Input: part model. Units: mm. Frame: model coordinates. A direction names the side the tool comes from. Give positions to 0.01 mm unless a question says otherwise; leave off trailing zeros. Write each loop counter-clockwise with the first axis right and the second up, starting at its lowest first coordinate (ties: lowest second). Pieces come first, ordered by that corner, then holes.
```python
from build123d import *

# Parameters (mm, degrees)
F0_W           = 80
F0_H           = 50
F0_R           = 19
F0_R_2         = 11
F1_DEPTH       = 15
F2_W           = 1
F2_H           = 15
F3_DEPTH       = 25
F5_D           = 5.5
F5_DEPTH       = 18
F5_CBORE_D     = 10
F5_CBORE_DEPTH = 5
F5_TIP         = 1.6523667023
F7_D           = 5.5
F7_DEPTH       = 15
F7_TIP         = 1.6523667023
F9_D           = 5.5
F9_DEPTH       = 15
F9_TIP         = 1.6523667023
F11_D          = 5.5
F11_DEPTH      = 15
F11_TIP        = 1.6523667023
F13_D          = 5.5
F13_DEPTH      = 10
F13_TIP        = 1.6523667023


with BuildPart() as f1:
    # F0 (on Top) → F1 (new body)
    with BuildSketch(Plane.XY):
        Rectangle(F0_W, F0_H)
        with Locations((-16, 0)):
            Circle(F0_R, mode=Mode.SUBTRACT)
        with Locations((24, 0)):
            Circle(F0_R_2, mode=Mode.SUBTRACT)
    extrude(amount=F1_DEPTH)

    # F2 (on face) → F3 (cut)
    with BuildSketch(Plane.XY.offset(15)):
        with Locations((23.5, -17.5)):
            Rectangle(F2_W, F2_H)
    extrude(amount=-F3_DEPTH, mode=Mode.SUBTRACT)

    # F5
    with Locations(Plane.YZ.offset(40)):
        with Locations((-17, 7.5)):
            CounterBoreHole(F5_D / 2, F5_CBORE_D / 2, F5_CBORE_DEPTH, depth=F5_DEPTH)
            with Locations((0, 0, -(F5_DEPTH + F5_TIP / 2))):  # 118° drill point
                Cone(0, F5_D / 2, F5_TIP, mode=Mode.SUBTRACT)

    # F7
    with Locations(Plane.YZ.offset(23)):
        with Locations((-17, 7.5)):
            Hole(F7_D / 2, depth=F7_DEPTH)
            with Locations((0, 0, -(F7_DEPTH + F7_TIP / 2))):  # 118° drill point
                Cone(0, F7_D / 2, F7_TIP, mode=Mode.SUBTRACT)

    # F9
    with Locations(Plane.XZ.offset(25)):
        with Locations((-16, 7.5)):
            Hole(F9_D / 2, depth=F9_DEPTH)
            with Locations((0, 0, -(F9_DEPTH + F9_TIP / 2))):  # 118° drill point
                Cone(0, F9_D / 2, F9_TIP, mode=Mode.SUBTRACT)

    # F11
    with Locations(Plane(origin=(-40, 0, 0), x_dir=(0, -1, 0), z_dir=(-1, 0, 0))):
        with Locations((0, 7.5)):
            Hole(F11_D / 2, depth=F11_DEPTH)
            with Locations((0, 0, -(F11_DEPTH + F11_TIP / 2))):  # 118° drill point
                Cone(0, F11_D / 2, F11_TIP, mode=Mode.SUBTRACT)

    # F13
    with Locations(Plane(origin=(0, 25, 0), x_dir=(-1, 0, 0), z_dir=(0, 1, 0))):
        with Locations((-32, 7.5), (-12, 7.5)):
            Hole(F13_D / 2, depth=F13_DEPTH)
            with Locations((0, 0, -(F13_DEPTH + F13_TIP / 2))):  # 118° drill point
                Cone(0, F13_D / 2, F13_TIP, mode=Mode.SUBTRACT)


solid = f1.part
```
Q1. Section B-B, the plane z = 1. Return the cut outline in (x, y), then the cut area to 3 significant figures.
Q2. Pin query (flat end, axial travel): pin 1 (6 mm diameter, centred on y = -16.5, z = 8, fed in from +X). Return the tip coordinate at first contact, or that it passes through.
Q3. Section A-A, the plane x = -16. Return the cut outline in (y, z), then the cut area to 3 significant figures.
Q4. Access query for faces 1 (the flat face through (-1, 25, 7)), 2 (the cylindrical face through (-13.818, -21.857, 5.827)), 3 (the cylindrical face through (-37.361, -0.596, 4.815)), 4 (the cylindrical face through (13.27, 19.93, 5.06)), 5 (the cylindrical face through (29.423, -14.818, 5.827)). Directions: +Z, -Z, +X, -X, +Y, -Y. A direction counts if a zero-diameter tool reaches every point of the face in a straight line with its end or side. Return the directions, or none.
Q5. Section D-D, the plane x = 20. Return the cut outline in (y, z), then the cut area to 3 significant figures.
Q6. Material intervals for line 1 along X through (y, z) = (20.5, 7.5); line 2 along X through (y, z) = (0, 4); line 3 along Z through (x, y) = (17, -17), sorted ascending.
Q7. Mould query, pull axis Z, two halves, no side actions, for faces 6 (the cylindrical face through (37.535, -20.685, 10.879)), 7 (the flat face through (8, 0, 15)), 8 (the flat face through (23, -20, 6)). Classes: +Z half, -Z half, draft (parallel to the pull), parting line (faces both ways), or undercut.
Q8. Section C-C, the plane y = 17. Return the cut outline in (x, z).
Solutions:
1. outline: (-40, -25) - (23, -25) - (23, -10.95) arc R11 cw (long way) to (24, -11) - (24, -25) - (40, -25) - (40, 25) - (-40, 25) - close; hole circle Ø38 at (-16, 0)
1. area: 2,470 mm2
2. pin 1: stops at x = 35
3. outline: (-25, 0) - (-19, 0) - (-19, 4.75) - (-25, 4.75) - close; (-25, 10.25) - (-19, 10.25) - (-19, 15) - (-25, 15) - close; (19, 0) - (25, 0) - (25, 15) - (19, 15) - close
3. area: 147 mm2
4. face 1: +Z, -Z, +X, -X, +Y
4. face 2: -Y
4. face 3: -X
4. face 4: +Y
4. face 5: +X
5. outline: (-25, 0) - (-10.25, 0) - (-10.25, 15) - (-25, 15) - close; (10.25, 0) - (25, 0) - (25, 15) - (10.25, 15) - close; hole circle Ø5.5 at (-17, 7.5)
5. area: 419 mm2
6. line 1: x = -40 to 9.25, 14.75 to 29.25, 34.75 to 40
6. line 2: x = -40 to -35, 3 to 13, 35 to 40
6. line 3: z = 0 to 4.75, 10.25 to 15
7. face 6: undercut
7. face 7: +Z half
7. face 8: draft
8. outline: (-40, 0) - (-24.49, 0) - (-24.49, 15) - (-40, 15) - close; (-7.51, 0) - (40, 0) - (40, 15) - (-7.51, 15) - close; hole circle Ø5.5 at (12, 7.5); hole circle Ø5.5 at (32, 7.5)
